Model file for the job. Use its own axes, mm. Face numbers are marked on the shaded views. A direction names the side the tool comes from. Round coordinates to 2 decimals unless told otherwise and drop trailing zeros. Loops run counter-clockwise (first coordinate to the right, second up) from the corner with the lowest first, then second, coordinate; pieces in that order, holes last. Notation, with made-up numbers: M 58,66 L 70,66 A24 cw 70,95 Z; hole C -34,15 d11. An arc over 180 degrees is marked long. Use a Markdown table: item, result. Add a question column.
Item 1: Saw through at C-C on x = 23. Write the cut outline in (y, z).
Item 2: Saw through at B-B on y = 20. Write the cut outline in (x, z), then the cut area to 3 significant figures.
Item 3: Pin check, flat tips, straight feed: P1, Ø12, axis at x = 14, z = -28, coming from the +Y side; P2, Ø6.5, axis at y = 20, z = -12.5, coming from the +X side; P3, Ø12.5, axis at y = 20, z = -37.5, coming from the +X side. Stop position of each tip, or through.
Item 4: Saw through at A-A on z = -37.5. Write the cut outline in (x, y).
Item 5: Wall check: L1, parallel to Y at x = 0.95, z = -37.5; L2, parallel to Y at x = 15, z = -30. Give the ranges that are in metal, low to high. Write a range as from..to.
Item 6: Tool access for the marked faces 1 and 2: list every direction of +Z, -Z, +X, -X, +Y, -Y with a clear straight run to the whole face (end or side of a thin tool).
Item 7: Saw through at D-D on z = -10. Write the cut outline in (x, y).
```python
from build123d import *

# Parameters (mm, degrees)
BOSS_EXTRUDE1_DEPTH = 50
SKETCH2_R           = 5.5
CUT_EXTRUDE1_DEPTH  = 70.057946682
SKETCH3_W           = 5
SKETCH3_H           = 5
CUT_EXTRUDE2_DEPTH  = 50


with BuildPart() as part:
    # Sketch1 → Boss-Extrude1 (new body)
    with BuildSketch(Plane.XY):
        Polygon((0, 4.805194805), (0, 0), (4.805194805, 0), (30, 0), (30, 2.5), (2.5, 2.5), (2.5, 37), (0, 37), align=None)
    extrude(amount=-BOSS_EXTRUDE1_DEPTH)

    # Sketch2 → Cut-Extrude1 (cut, through all)
    with BuildSketch(Plane.ZY):
        with Locations((-37.5, 20)):
            Circle(SKETCH2_R)
        with Locations((-12.5, 20)):
            Circle(SKETCH2_R)
    extrude(amount=-CUT_EXTRUDE1_DEPTH, mode=Mode.SUBTRACT)

    # Sketch3 → Cut-Extrude2 (cut)
    with BuildSketch(Plane.XZ):
        with Locations((21.5, -8.5)):
            Rectangle(SKETCH3_W, SKETCH3_H)
        with Locations((21.5, -41.5)):
            Rectangle(SKETCH3_W, SKETCH3_H)
    extrude(amount=-CUT_EXTRUDE2_DEPTH, mode=Mode.SUBTRACT)


solid = part.part
```
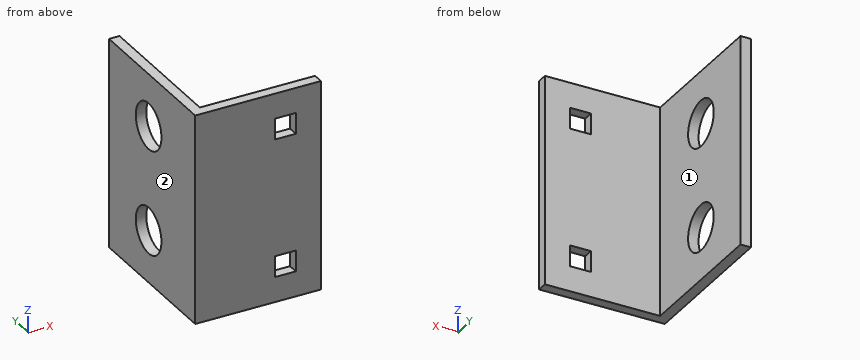
Entries:
| question | item | result |
|---|---|---|
| 1 | outline | M 0,-50 L 2.5,-50 L 2.5,-44 L 0,-44 Z; M 0,-39 L 2.5,-39 L 2.5,-11 L 0,-11 Z; M 0,-6 L 2.5,-6 L 2.5,0 L 0,0 Z |
| 2 | outline | M 0,-50 L 2.5,-50 L 2.5,-43 L 0,-43 Z; M 0,-32 L 2.5,-32 L 2.5,-18 L 0,-18 Z; M 0,-7 L 2.5,-7 L 2.5,0 L 0,0 Z |
| 2 | area | 70.0 mm2 |
| 3 | P1 | y = 2.5 |
| 3 | P2 | through |
| 3 | P3 | x = 2.5 |
| 4 | outline | M 0,0 L 30,0 L 30,2.5 L 2.5,2.5 L 2.5,14.5 L 0,14.5 Z; M 0,25.5 L 2.5,25.5 L 2.5,37 L 0,37 Z |
| 5 | L1 | 0..14.5, 25.5..37 |
| 5 | L2 | 0..2.5 |
| 6 | face 1 | +Z, -Z, +X, +Y |
| 6 | face 2 | +Z, -Z, -X, +Y, -Y |
| 7 | outline | M 0,0 L 19,0 L 19,2.5 L 2.5,2.5 L 2.5,15.1 L 0,15.1 Z; M 0,24.9 L 2.5,24.9 L 2.5,37 L 0,37 Z; M 24,0 L 30,0 L 30,2.5 L 24,2.5 Z |
